from build123d import *

# Parameters (mm, degrees)
SKETCH1_R               = 4.2164
MOUNTING_PLATE_MP_DEPTH = 5.08
WHEEL_SUPPORT_1_DEPTH   = 5.08
FILLET1_R               = 2.54
FILLET2_R               = 0.635


with BuildPart() as part:
    # Sketch1 → Mounting Plate (MP) (new body)
    with BuildSketch(Plane(origin=(0, 0, 0), x_dir=(1, 0, 0), z_dir=(0, 1, 0))):
        with BuildLine():
            Line((-40.132, 38.1), (40.132, 38.1))
            ThreePointArc((40.132, 38.1), (47.675415142, 34.975415142), (50.8, 27.432))
            Line((50.8, 27.432), (50.8, -27.432))
            ThreePointArc((50.8, -27.432), (47.675415142, -34.975415142), (40.132, -38.1))
            Line((40.132, -38.1), (-40.132, -38.1))
            ThreePointArc((-40.132, -38.1), (-47.675415142, -34.975415142), (-50.8, -27.432))
            Line((-50.8, -27.432), (-50.8, 27.432))
            ThreePointArc((-50.8, 27.432), (-47.675415142, 34.975415142), (-40.132, 38.1))
        make_face()
        with Locations((38.2143, 22.3393)):
            Circle(SKETCH1_R, mode=Mode.SUBTRACT)
        with Locations((-38.2143, 22.3393)):
            Circle(SKETCH1_R, mode=Mode.SUBTRACT)
        with Locations((-38.2143, -22.3393)):
            Circle(SKETCH1_R, mode=Mode.SUBTRACT)
        with Locations((38.2143, -22.3393)):
            Circle(SKETCH1_R, mode=Mode.SUBTRACT)
    extrude(amount=MOUNTING_PLATE_MP_DEPTH)

    # Sketch2 → MP Bearing Retainer (revolve)
    with BuildSketch(Plane.XY):
        with BuildLine():
            Line((0, 9.652), (-29.893008834, 9.652))
            ThreePointArc((-29.893008834, 9.652), (-34.590292304, 8.431881878), (-38.1, 5.08))
            Line((-38.1, 5.08), (0, 5.08))
            Line((0, 5.08), (0, 9.652))
        make_face()
    revolve(axis=Axis((0, 5.08, 0), (0, 1, 0)))

    # Sketch3 → Caster Wheel Base (revolve)
    with BuildSketch(Plane.XY):
        Polygon((0, 9.652), (-6.35, 9.652), (-6.35, 10.922), (-29.972, 10.922), (-29.972, 13.716), (0, 13.716), align=None)
    revolve(axis=Axis((0, 13.716, 0), (0, -1, 0)))

    # Sketch7 → Wheel Support 1 (add)
    with BuildSketch(Plane.ZY.offset(-21.209)):
        with BuildLine():
            Line((10.072633417, 97.849532267), (21.177797407, 13.716))
            Line((21.177797407, 13.716), (-21.177797407, 13.716))
            Line((-21.177797407, 13.716), (-10.072633417, 97.849532267))
            ThreePointArc((-10.072633417, 97.849532267), (0, 106.68), (10.072633417, 97.849532267))
        make_face()
    wheel_support_1 = extrude(amount=WHEEL_SUPPORT_1_DEPTH)

    # Wheel Support 2: Wheel Support 1 across plane
    add(wheel_support_1.mirror(Plane.ZY))

    # Sketch9 → Revolve3 (revolve)
    with BuildSketch(Plane(origin=(0, 96.52, 0), x_dir=(1, 0, 0), z_dir=(0, 1, 0))):
        with BuildLine():
            Line((-16.129, 0), (16.129, 0))
            Line((16.129, 0), (16.129, 12.574245218))
            ThreePointArc((16.129, 12.574245218), (16.122819325, 12.699387993), (16.104337458, 12.823312709))
            Line((16.104337458, 12.823312709), (15.875, 13.97))
            Line((15.875, 13.97), (15.875, 63.5))
            Line((15.875, 63.5), (-15.875, 63.5))
            Line((-15.875, 63.5), (-15.875, 13.97))
            Line((-15.875, 13.97), (-16.104337458, 12.823312709))
            ThreePointArc((-16.104337458, 12.823312709), (-16.122819325, 12.699387993), (-16.129, 12.574245218))
            Line((-16.129, 12.574245218), (-16.129, 0))
        make_face()
    revolve(axis=Axis((-16.129, 96.52, 0), (1, 0, 0)))

    # Fillet1
    fillet1_edges = [part.edges().sort_by_distance(p)[0] for p in [
        (15.875, 96.52, 63.5),
        (-15.875, 96.52, 63.5),
    ]]
    fillet(fillet1_edges, radius=FILLET1_R)

    # Fillet2
    fillet2_edges = [part.edges().sort_by_distance(p)[0] for p in [
        (29.972, 10.922, 0),
    ]]
    fillet(fillet2_edges, radius=FILLET2_R)


solid = part.part
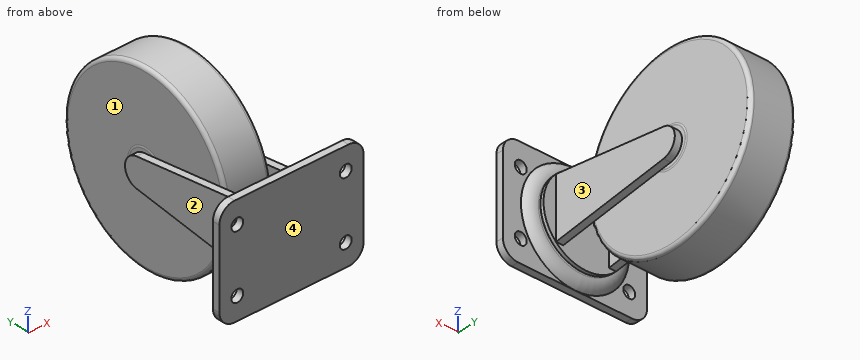
Read the model definition and answer for the solid it produces. Units are mm, in the model's axes. Face numbers are marked on the shaded views. Round coordinates to 2 decimals unless told otherwise and drop trailing zeros. Order: outer loops, then holes, each group sorted by start corner. A loop starts at its lowest first (then second) coordinate and runs counter-clockwise, first axis right, second up.
1) Flat-ended cylindrical pins translate along their axes: pin 1 (8 mm diameter, centred on x = 9, z = -12, fed in from +Y); pin 2 (2.5 mm diameter, centred on x = -24.5, z = -5, fed in from +Y); pin 3 (10 mm diameter, centred on x = 25, y = 46, fed in from +Z). Find the tip coordinate at first contact, or state that the pin passes through.
2) Straight lines are drawn through the part: L1, parallel to X at y = 93, z = -44 (3 decimals); L2, parallel to Y at x = -25, z = -5.5; L3, parallel to Y at x = -34, z = 25. For each, find the intervals that lie inside material, in ascending order.
3) The mould has two halves that part along X. Classify the marked faces 1, 2, 3 and 4: released by +X, released by -X, zero draft, split by the parting line, or undercut.
4) The part is cut by section A-A on y = 18.5. Write down the section's boundary in (x, z), plus the area to 3 significant figures.
5) The part is cut by section B-B on y = 50. Give the number of separate pieces and of enclosed holes in the cut face, plus the area to 3 significant figures.
Resolved:
1. pin 1: stops at y = 159.51
1. pin 2: stops at y = 13.72
1. pin 3: stops at z = 17.35
2. L1: x = -15.875 to 15.875
2. L2: y = 0 to 9.65, 10.92 to 13.72
2. L3: y = 0 to 5.08
3. face 1: undercut
3. face 2: released by -X
3. face 3: released by +X
3. face 4: zero draft
4. outline: (-21.21, -20.55) - (-16.13, -20.55) - (-16.13, 20.55) - (-21.21, 20.55) - close; (16.13, -20.55) - (21.21, -20.55) - (21.21, 20.55) - (16.13, 20.55) - close
4. area: 418 mm2
5. separate pieces: 3
5. enclosed holes: 0
5. area: 3,070 mm2
